Verification items for this drawing (mm, ordinates from the low corner). A direction names the side the tool comes from. Round coordinates to 2 decimals unless told otherwise and drop trailing zeros. Loops run counter-clockwise (first coordinate to the right, second up) from the corner with the lowest first, then second, coordinate; pieces in that order, holes last. Notation, with made-up numbers: M 74,16.5 L 78,16.5 A7 cw 78,26.5 Z; hole C 24.25,16.25 d10. An arc over 180 degrees is marked long. Use one line per item in the form item = value. Start each with the question number.
1. Cross-section at B-B (z = 29). Record the boundary of the cut face in (x, y), then the cut area to 3 significant figures.
2. Draft check along Y on the marked faces 1 and 2. Enter one of: pulls with the +Y half, pulls with the -Y half, needs draft (parallel to the pull), parting line crosses it, or undercut.
3. Set-up check for the marked faces 3 and 4: record each of +Z, -Z, +X, -X, +Y, -Y from which the full face is reachable in a straight line by a thin tool's end or side.
4. Material ranges on line 1 (Y direction, x = 26, z = 36) (1 decimal); line 2 (X direction, y = 16.5, z = 35); line 3 (Y direction, x = 33.5, z = 14.5) (1 decimal), recorded low to high.
5. Cross-section at A-A (z = 21.5). Record the boundary of the cut face in (x, y).
6. Go/stop test with flat-tipped pins: pin 1 (6 mm diameter, centred on x = 13.5, z = 8, fed in from +Y) (1 decimal); pin 2 (6 mm diameter, centred on x = 8.5, z = 38, fed in from -Y) (1 decimal); pin 3 (8 mm diameter, centred on y = 10.5, z = 41, fed in from -X). Record where each tip stops, or that it passes through.
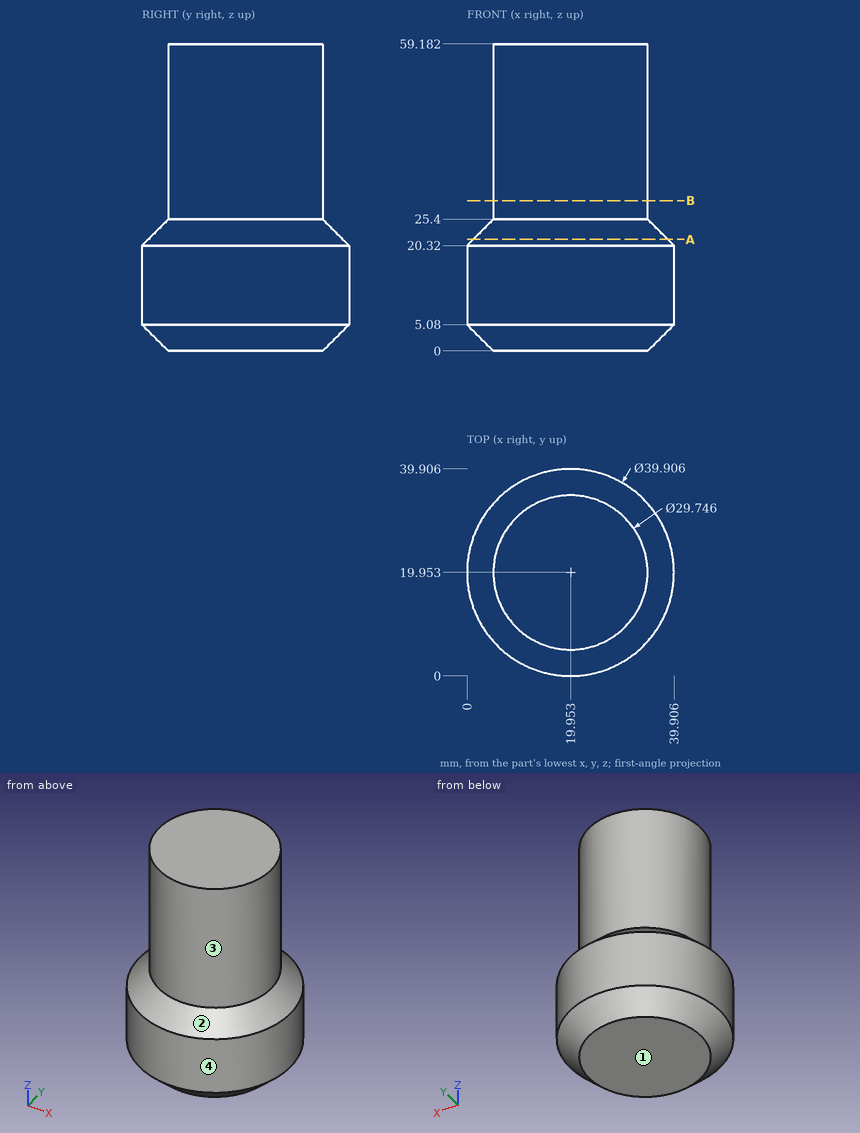
Reported:
q1.outline = C 19.95,19.95 d29.75
q1.area = 695 mm²
q2.face_1 = needs draft
q2.face_2 = parting line crosses it
q3.face_3 = +Z
q3.face_4 = +Z, -Z
q4.line_1 = 6.4 to 33.5
q4.line_2 = 5.49 to 34.42
q4.line_3 = 5.3 to 34.6
q5.outline = C 19.95,19.95 d37.55
q6.pin_1 = 39.6
q6.pin_2 = 7.7
q6.pin_3 = 6.12
